```python
from build123d import *

# Parameters (mm, degrees)
SKETCH_4_R        = 50
EXTRUDE_1_DEPTH   = 200
MOVE_BODY_1_ANGLE = 10


with BuildPart() as part:
    # 放样1: read off the stored shape, not the designer's step
    # 放样1: loft between two sections, ruled curve by curve
    loft_1_from = [
        Edge.make_bspline([(666.999999998, 0, 1000), (663.799637222, -0.604724548, 1000), (656.220345397, -2.022885982, 1000), (645.979516294, -3.898542902, 1000), (635.247963028, -5.826243875, 1000), (624.819981281, -7.662584434, 1000), (614.198521539, -9.496021813, 1000), (599.972074061, -11.904629718, 1000), (582.430830371, -14.787740297, 1000), (561.135044503, -18.155812197, 1000), (539.946417674, -21.377647562, 1000), (518.671869989, -24.487157927, 1000), (497.416172992, -27.468442034, 1000), (476.123475264, -30.32944244, 1000), (454.824744619, -33.062783586, 1000), (433.50415239, -35.666455969, 1000), (412.170012578, -38.132804161, 1000), (390.818267621, -40.453999041, 1000), (369.450759947, -42.619108718, 1000), (348.066446531, -44.61511771, 1000), (326.665801057, -46.426441856, 1000), (305.24879013, -48.034169355, 1000), (283.816053008, -49.416509673, 1000), (262.368394512, -50.54750092, 1000), (240.907772126, -51.396721383, 1000), (219.436549528, -51.928303079, 1000), (201.539164161, -52.070683511, 1000), (187.221095545, -51.978850226, 1000), (176.483975584, -51.799236258, 1000), (165.749412964, -51.500531623, 1000), (155.01932189, -51.073159695, 1000), (144.295530458, -50.506856143, 1000), (133.580710906, -49.789673503, 1000), (122.878050961, -48.907360236, 1000), (112.192125096, -47.843447663, 1000), (101.527781752, -46.578273412, 1000), (90.892670861, -45.089586686, 1000), (80.294429011, -43.348017915, 1000), (69.750642268, -41.316102027, 1000), (59.27225592, -38.947539372, 1000), (50.626877349, -36.641275533, 1000), (43.777772332, -34.54819846, 1000), (38.687572512, -32.840917397, 1000), (33.65117684, -30.975832975, 1000), (28.686664939, -28.92949158, 1000), (23.813093939, -26.671460223, 1000), (19.064458401, -24.161974773, 1000), (14.487509708, -21.346794417, 1000), (10.161987345, -18.156904498, 1000), (6.218399789, -14.494122288, 1000), (2.887973837, -10.257639927, 1000), (0.554665428, -5.36560271, 1000), (-0.00056538, -1.793819625, 1000), (0, 0, 1000)], [0, 0, 0, 0, 0.015625, 0.03125, 0.046875, 0.0625, 0.078125, 0.09375, 0.125, 0.15625, 0.1875, 0.21875, 0.25, 0.28125, 0.3125, 0.34375, 0.375, 0.40625, 0.4375, 0.46875, 0.5, 0.53125, 0.5625, 0.59375, 0.625, 0.65625, 0.6875, 0.703125, 0.71875, 0.734375, 0.75, 0.765625, 0.78125, 0.796875, 0.8125, 0.828125, 0.84375, 0.859375, 0.875, 0.890625, 0.90625, 0.9140625, 0.921875, 0.9296875, 0.9375, 0.9453125, 0.953125, 0.9609375, 0.96875, 0.9765625, 0.984375, 0.9921875, 1, 1, 1, 1], 3),
        Edge.make_bspline([(0, 0, 1000), (-0.00056538, 1.793819625, 1000), (0.554665457, 5.365602719, 1000), (2.887973782, 10.257639911, 1000), (6.218399893, 14.494122319, 1000), (10.16198715, 18.156904441, 1000), (14.487510113, 21.346794535, 1000), (19.064457581, 24.161974532, 1000), (23.813095456, 26.671460667, 1000), (28.686661745, 28.929490645, 1000), (33.651182789, 30.975834716, 1000), (38.687562847, 32.840914568, 1000), (43.77777737, 34.548199936, 1000), (50.627004326, 36.641312682, 1000), (59.272176198, 38.947516048, 1000), (69.75068889, 41.316115667, 1000), (80.294402937, 43.348010287, 1000), (90.892684893, 45.089590791, 1000), (101.527774389, 46.578271259, 1000), (112.192129243, 47.843448873, 1000), (122.878048588, 48.907359547, 1000), (133.580712133, 49.789673852, 1000), (144.295529784, 50.506855964, 1000), (155.019322303, 51.073159781, 1000), (165.7494126, 51.500531586, 1000), (176.483976098, 51.799236258, 1000), (187.221094044, 51.978850255, 1000), (201.539174789, 52.070683467, 1000), (219.436542978, 51.928303134, 1000), (240.907775179, 51.396721346, 1000), (262.368393037, 50.54750093, 1000), (283.816053471, 49.416509703, 1000), (305.248790507, 48.034169261, 1000), (326.665799717, 46.426442055, 1000), (348.066449966, 44.615117246, 1000), (369.450753442, 42.619109596, 1000), (390.818280118, 40.453997321, 1000), (412.169989323, 38.132807449, 1000), (433.504199323, 35.666449175, 1000), (454.824640648, 33.062798963, 1000), (476.123661756, 30.329414262, 1000), (497.415809346, 27.468498036, 1000), (518.672557556, 24.487049873, 1000), (539.945247415, 21.377835197, 1000), (561.137421083, 18.155424744, 1000), (582.426549093, 14.788450701, 1000), (599.977986088, 11.903627109, 1000), (614.193135953, 9.496953161, 1000), (624.809385208, 7.66440837, 1000), (635.248408041, 5.826192456, 1000), (645.979996559, 3.898441222, 1000), (656.220005166, 2.022955598, 1000), (663.799637221, 0.604724548, 1000), (666.999999998, 0, 1000)], [0, 0, 0, 0, 0.0078125, 0.015625, 0.0234375, 0.03125, 0.0390625, 0.046875, 0.0546875, 0.0625, 0.0703125, 0.078125, 0.0859375, 0.09375, 0.109375, 0.125, 0.140625, 0.15625, 0.171875, 0.1875, 0.203125, 0.21875, 0.234375, 0.25, 0.265625, 0.28125, 0.296875, 0.3125, 0.34375, 0.375, 0.40625, 0.4375, 0.46875, 0.5, 0.53125, 0.5625, 0.59375, 0.625, 0.65625, 0.6875, 0.71875, 0.75, 0.78125, 0.8125, 0.84375, 0.875, 0.90625, 0.921875, 0.9375, 0.953125, 0.96875, 0.984375, 1, 1, 1, 1], 3),
    ]
    loft_1_to = [
        Edge.make_bspline([(667, 0, 0), (663.787937121, -0.778122232, 0), (656.200450193, -2.598380354, 0), (645.874703604, -5.022316958, 0), (635.152751042, -7.491793756, 0), (624.5656651, -9.880168768, 0), (613.932901468, -12.233182769, 0), (599.674290652, -15.325646654, 0), (581.992397773, -19.049903866, 0), (560.57943939, -23.387245223, 0), (539.221710022, -27.546205859, 0), (517.787201902, -31.556421716, 0), (496.348785222, -35.404191447, 0), (474.869299834, -39.09532252, 0), (453.369610223, -42.622057623, 0), (431.838824667, -45.980159867, 0), (410.283069511, -49.159666954, 0), (388.699054607, -52.149437047, 0), (367.088216437, -54.934513775, 0), (345.449452769, -57.497118306, 0), (323.783329406, -59.815457029, 0), (302.089797679, -61.863709181, 0), (280.370013167, -63.611758836, 0), (258.625333152, -65.023318773, 0), (236.859716284, -66.056526685, 0), (215.07684211, -66.660710105, 0), (196.918876775, -66.757547051, 0), (182.392533714, -66.55498137, 0), (171.501404926, -66.251902277, 0), (160.617518552, -65.786531136, 0), (149.742132912, -65.14508538, 0), (138.876506323, -64.313782442, 0), (128.032113187, -63.275126167, 0), (117.209580934, -62.009887151, 0), (106.420382287, -60.495066539, 0), (95.672322051, -58.704678377, 0), (84.980781239, -56.605895334, 0), (74.36207887, -54.160061058, 0), (63.842374932, -51.318325944, 0), (53.456401835, -48.016417607, 0), (44.957838639, -44.813840559, 0), (38.292062891, -41.923609068, 0), (33.377232896, -39.572370085, 0), (28.56486913, -37.018085304, 0), (23.883463681, -34.231740425, 0), (19.36150864, -31.18432115, 0), (15.060271723, -27.837579504, 0), (11.041020644, -24.153267514, 0), (7.406069775, -20.084935176, 0), (4.290999374, -15.600598491, 0), (1.871979479, -10.701125876, 0), (0.340748863, -5.445801038, 0), (-0.000762063, -1.818923188, 0), (0, 0, 0)], [0, 0, 0, 0, 0.015625, 0.03125, 0.046875, 0.0625, 0.078125, 0.09375, 0.125, 0.15625, 0.1875, 0.21875, 0.25, 0.28125, 0.3125, 0.34375, 0.375, 0.40625, 0.4375, 0.46875, 0.5, 0.53125, 0.5625, 0.59375, 0.625, 0.65625, 0.6875, 0.703125, 0.71875, 0.734375, 0.75, 0.765625, 0.78125, 0.796875, 0.8125, 0.828125, 0.84375, 0.859375, 0.875, 0.890625, 0.90625, 0.9140625, 0.921875, 0.9296875, 0.9375, 0.9453125, 0.953125, 0.9609375, 0.96875, 0.9765625, 0.984375, 0.9921875, 1, 1, 1, 1], 3),
        Edge.make_bspline([(0, 0, 0), (-0.000762063, 1.818923188, 0), (0.340748548, 5.445800771, 0), (1.871980086, 10.701126391, 0), (4.290998372, 15.600597641, 0), (7.406071183, 20.084936371, 0), (11.041021844, 24.15326852, 0), (15.060236322, 27.837549592, 0), (19.361493058, 31.184307985, 0), (23.883478049, 34.231752566, 0), (28.564877292, 37.018092199, 0), (33.377225985, 39.572364244, 0), (38.292059332, 41.923606062, 0), (44.957845322, 44.81384621, 0), (53.456396907, 48.016413426, 0), (63.842377593, 51.318328228, 0), (74.36207734, 54.160059689, 0), (84.980781846, 56.605896032, 0), (95.6723223, 58.704678198, 0), (106.420381084, 60.495066274, 0), (117.209583402, 62.009887926, 0), (128.03211035, 63.275124839, 0), (138.876497485, 64.313783504, 0), (149.742260365, 65.145092619, 0), (160.617583681, 65.786535028, 0), (171.501366862, 66.251900805, 0), (182.392509333, 66.554980024, 0), (196.91891222, 66.75754823, 0), (215.076816077, 66.660709555, 0), (236.859730532, 66.056526855, 0), (258.625324823, 65.023318727, 0), (280.370017887, 63.611758862, 0), (302.089795835, 61.863709105, 0), (323.783329573, 59.815457216, 0), (345.449454995, 57.497117841, 0), (367.088211422, 54.934514671, 0), (388.699064902, 52.149435238, 0), (410.283049885, 49.15967045, 0), (431.83886648, 45.980152247, 0), (453.369533879, 42.622071814, 0), (474.869445862, 39.095294769, 0), (496.348540372, 35.404238832, 0), (517.787684284, 31.556326568, 0), (539.220784537, 27.546391723, 0), (560.581135329, 23.386898456, 0), (581.988814982, 19.050650465, 0), (599.680611516, 15.324311348, 0), (613.932935101, 12.233157769, 0), (624.565379788, 9.880240812, 0), (635.152932724, 7.491748581, 0), (645.874603859, 5.02234186, 0), (656.200501376, 2.598367496, 0), (663.787937121, 0.778122232, 0), (667, 0, 0)], [0, 0, 0, 0, 0.0078125, 0.015625, 0.0234375, 0.03125, 0.0390625, 0.046875, 0.0546875, 0.0625, 0.0703125, 0.078125, 0.0859375, 0.09375, 0.109375, 0.125, 0.140625, 0.15625, 0.171875, 0.1875, 0.203125, 0.21875, 0.234375, 0.25, 0.265625, 0.28125, 0.296875, 0.3125, 0.34375, 0.375, 0.40625, 0.4375, 0.46875, 0.5, 0.53125, 0.5625, 0.59375, 0.625, 0.65625, 0.6875, 0.71875, 0.75, 0.78125, 0.8125, 0.84375, 0.875, 0.90625, 0.921875, 0.9375, 0.953125, 0.96875, 0.984375, 1, 1, 1, 1], 3),
    ]
    loft_1 = Solid(Shell([*[Face.make_surface_from_curves(loft_1_from[k], loft_1_to[k]) for k in range(2)], Face(Wire(loft_1_from)), Face(Wire(loft_1_to))]))
    add(loft_1)

    # 草图4 → 凸台-拉伸1 (add)
    with BuildSketch(Plane(origin=(0, 0, 0), x_dir=(-1, 0, 0), z_dir=(0, 0, -1))):
        with Locations((-200, 0)):
            Circle(SKETCH_4_R)
    extrude(amount=EXTRUDE_1_DEPTH)


with BuildPart() as part_1:
    # Move Body 1: moved
    add(part.part.rotate(Axis((333.49958875, 7.784e-06, 0), (0, 0, -1)), MOVE_BODY_1_ANGLE))


solid = part_1.part
```
Geometry check sheet. Reference: the model listing, model coordinates, mm. A direction names the side the tool comes from. Coordinates: 2 decimals unless noted, no trailing zeros.
Q1. Tool access check on faces 1 (the face through (203, 24, -200)), 2 (the face through (244.19, 50.06, -98.6)). Record the directions out of +Z, -Z, +X, -X, +Y, -Y that give a thin tool (end or side, any length) a straight path to the whole face; none if there is none.
Reply:
face 1: -Z, +X, -X, +Y, -Y
face 2: -Z
Q2. Thickness scan on probe 1 along Z at (x, y) = (326.5, 13); probe 2 along X at (y, z) = (48, -8); probe 3 along X at (y, z) = (-22.5, -129.5). Record the ranges inside material, lowest first.
Reply:
probe 1: z = 0 to 1000
probe 2: x = 158.62 to 245.43
probe 3: x = 181.7 to 222.35
Q3. Depth check by flat-ended pin: pin 1 Ø6 at (y, z) = (22.5, -64.5) entering from +X; pin 2 Ø8 at (y, z) = (18, 322) entering from -X; pin 3 Ø1 at (x, z) = (206, 345.5) entering from +Y. Enter the tip coordinate at first touch or a pass-through.
Reply:
pin 1: stops at x = 252.03
pin 2: stops at x = 23.89
pin 3: stops at y = 85.13
